from build123d import *

# Parameters (mm, degrees)
SALIENTE_EXTRUIR1_DEPTH = 60
REDONDEO1_R             = 2
CROQUIS2_R              = 3.5
CORTAR_EXTRUIR1_DEPTH   = 60
CHAFL_N1_SIZE           = 1


with BuildPart() as part:
    # Croquis1 → Saliente-Extruir1 (new body)
    with BuildSketch(Plane.XY):
        Polygon((-16.031190476, -21.01547619), (-16.031190476, 0.81452381), (8.148809524, 0.81452381), (8.148809524, 30.81452381), (4.978809524, 30.81452381), (4.978809524, 3.98452381), (-19.201190476, 3.98452381), (-19.201190476, -21.01547619), align=None)
    extrude(amount=SALIENTE_EXTRUIR1_DEPTH)

    # Redondeo1
    redondeo1_edges = [part.edges().sort_by_distance(p)[0] for p in [
        (-19.201190476, 3.98452381, 30),
        (4.978809524, 3.98452381, 30),
        (8.148809524, 0.81452381, 30),
        (-16.031190476, 0.81452381, 30),
    ]]
    fillet(redondeo1_edges, radius=REDONDEO1_R)

    # Croquis2 → Cortar-Extruir1 (cut)
    with BuildSketch(Plane(origin=(8.148809524, 0, 0), x_dir=(0, 0, -1), z_dir=(1, 0, 0))):
        with Locations((-53, 18.81452381)):
            Circle(CROQUIS2_R)
        with Locations((-7, 18.81452381)):
            Circle(CROQUIS2_R)
    extrude(amount=-CORTAR_EXTRUIR1_DEPTH, mode=Mode.SUBTRACT)

    # Chaflán1
    chafl_n1_edges = [part.edges().sort_by_distance(p)[0] for p in [
        (-16.031190476, -11.10047619, 0),
        (-19.201190476, -21.01547619, 30),
        (4.978809524, 30.81452381, 30),
        (8.148809524, 30.81452381, 30),
        (-16.031190476, -21.01547619, 30),
        (6.563809524, 30.81452381, 60),
        (4.978809524, 18.39952381, 60),
        (-19.201190476, -9.51547619, 0),
        (-19.201190476, -9.51547619, 60),
        (-7.111190476, 3.98452381, 0),
        (8.148809524, 16.81452381, 0),
        (-3.941190476, 0.81452381, 0),
        (7.563023086, 1.400310247, 0),
        (-18.615404039, 3.398737372, 0),
        (-7.111190476, 3.98452381, 60),
        (-3.941190476, 0.81452381, 60),
        (8.148809524, 16.81452381, 60),
        (7.563023086, 1.400310247, 60),
        (-18.615404039, 3.398737372, 60),
        (4.393023086, 4.570310247, 0),
        (4.393023086, 4.570310247, 60),
        (-15.445404039, 0.228737372, 0),
        (-15.445404039, 0.228737372, 60),
        (-16.031190476, -11.10047619, 60),
        (4.978809524, 18.39952381, 0),
    ]]
    chamfer(chafl_n1_edges, length=CHAFL_N1_SIZE)


solid = part.part
Geometry check sheet. Reference: the model listing, model coordinates, mm. A direction names the side the tool comes from. Coordinates: 2 decimals unless noted, no trailing zeros. Loops run counter-clockwise (first coordinate to the right, second up) from the corner with the lowest first, then second, coordinate; pieces in that order, holes last. Notation, with made-up numbers: (61, 17) - (74, 17) arc R25 ccw to (74, 54) - close; hole circle Ø4 at (26, 64). An arc over 180 degrees is marked (long way). Use one line per item in the form item = value. Start each with the question number.
Item 1: Section check D-D, the plane y = -9. Enter the section's corners in (x, z).
Item 2: Section check A-A, the plane z = 53. Enter the section's corners in (x, y).
Item 3: Section check B-B, the plane x = -1. Enter the section's corners in (y, z).
Item 4: Tool access check on faces 4 (the face through (-4, 0.815, 30)), 5 (the face through (4.979, 18, 30)), 6 (the face through (-15.744, 0.49, 0.604)). Record the directions out of +Z, -Z, +X, -X, +Y, -Y that give a thin tool (end or side, any length) a straight path to the whole face; none if there is none.
Item 5: Gauge pin test, flat ends, axial feed: pin 1 (4 mm diameter, centred on x = 2, z = 20, fed in from +Y); pin 2 (6 mm diameter, centred on x = -1.5, z = 44, fed in from -Y); pin 3 (15 mm diameter, centred on y = -15, z = 19, fed in from +X). Record the tip position at first contact, or that the pin passes through.
Item 6: Thickness scan on probe 1 along Y at (x, z) = (6.3, 7); probe 2 along X at (y, z) = (-14, 30.5); probe 3 along X at (y, z) = (24, 48.5). Record the ranges inside material, lowest first.
Item 7: Section check C-C, the plane z = 21.5. Enter the section's corners in (x, y), and give its area (3 significant figures).
Item 8: Mould release check, pull along Z, two halves, no side actions. Record for faces 1 (the face through (6.586, 18.968, 56.497)), 2 (the face through (-18.177, 2.982, 59.604)), 3 (the face through (-18.177, 2.982, 0.396)): +Z half, -Z half, draft (parallel to the pull), parting line (faces both ways), or undercut.
Computed:
q1.outline = (-19.2, 1) - (-18.2, 0) - (-17.03, 0) - (-16.03, 1) - (-16.03, 59) - (-17.03, 60) - (-18.2, 60) - (-19.2, 59) - close
q2.outline = (-19.2, -20.02) - (-18.2, -21.02) - (-17.03, -21.02) - (-16.03, -20.02) - (-16.03, -1.19) arc R2 cw to (-14.03, 0.81) - (6.15, 0.81) arc R2 ccw to (8.15, 2.81) - (8.15, 15.31) - (4.98, 15.31) - (4.98, 5.98) arc R2 cw to (2.98, 3.98) - (-17.2, 3.98) arc R2 ccw to (-19.2, 1.98) - close; (4.98, 22.31) - (8.15, 22.31) - (8.15, 29.81) - (7.15, 30.81) - (5.98, 30.81) - (4.98, 29.81) - close
q3.outline = (0.81, 1) - (1.81, 0) - (2.98, 0) - (3.98, 1) - (3.98, 59) - (2.98, 60) - (1.81, 60) - (0.81, 59) - close
q4.face_4 = +Z, -Z, +X, -Y
q4.face_5 = +Z, -Z, -X, +Y
q4.face_6 = -Z, +X, -Y
q5.pin_1 = 4.26
q5.pin_2 = 0.81
q5.pin_3 = -16.03
q6.probe_1 = 0.82 to 15.31, 22.31 to 30.81
q6.probe_2 = -19.2 to -16.03
q6.probe_3 = 4.98 to 8.15
q7.outline = (-19.2, -20.02) - (-18.2, -21.02) - (-17.03, -21.02) - (-16.03, -20.02) - (-16.03, -1.19) arc R2 cw to (-14.03, 0.81) - (6.15, 0.81) arc R2 ccw to (8.15, 2.81) - (8.15, 29.81) - (7.15, 30.81) - (5.98, 30.81) - (4.98, 29.81) - (4.98, 5.98) arc R2 cw to (2.98, 3.98) - (-17.2, 3.98) arc R2 ccw to (-19.2, 1.98) - close
q7.area = 239 mm2
q8.face_1 = undercut
q8.face_2 = +Z half
q8.face_3 = -Z half
